The figure shows three views and two pictorial views of one solid part (mm, origin at its lowest corner). Answer the questions. Give positions to 0.01 mm unless a question says otherwise; leave off trailing zeros. Loops run counter-clockwise (first coordinate to the right, second up) from the corner with the lowest first, then second, coordinate; pieces in that order, holes last. Notation, with made-up numbers: (80.5, 26.25) - (101.5, 26.25) arc R12 ccw to (101.5, 44.25) - close; hole circle Ø6 at (63, 35.5). An arc over 180 degrees is marked (long way). Use CSV: the item, a comma, the result in double quotes.
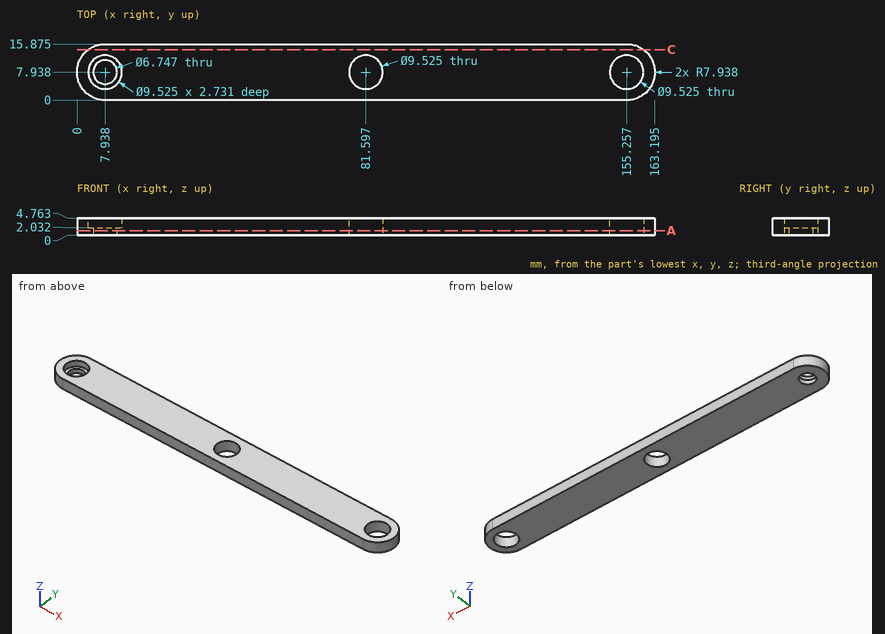
Item 1: Find the intervals of material crossed by line 1 (X direction, y = 7.75, z = 0.45) (1 decimal); line 2 (X direction, y = 9.5, z = 1.15) (1 decimal); line 3 (X direction, y = 14, z = 4.2) (1 decimal), in increasing order.
Determined:
line 1,"x = 0 to 4.6, 11.3 to 76.8, 86.4 to 150.5, 160 to 163.2"
line 2,"x = 0.2 to 4.9, 10.9 to 77.1, 86.1 to 150.8, 159.8 to 163"
line 3,"x = 2.8 to 160.4"
Item 2: A cutting plane is placed at A-A on z = 1.25. Determine the outline of the cut face in (x, y) (1 decimal).
Determined:
outline,"(7.9, 0) - (155.3, 0) arc R7.9 ccw to (155.3, 15.9) - (7.9, 15.9) arc R7.9 ccw to start; hole circle Ø6.7 at (7.9, 7.9); hole circle Ø9.5 at (81.6, 7.9); hole circle Ø9.5 at (155.3, 7.9)"
Item 3: A cutting plane is placed at C-C on y = 14.25. Determine the outline of the cut face in (x, z) (1 decimal).
Determined:
outline,"(3.1, 0) - (160.1, 0) - (160.1, 4.8) - (3.1, 4.8) - close"
Item 4: Given P1, Ø2, axis at y = 5, z = 1.5, coming from the +X side (1 decimal), flat-ended and moving along its own axis, determine where the tip first touches the part or whether it passes through.
Determined:
P1,"stops at x = 163"
